CAD build for the part. Positions are in the model's coordinates, mm. A direction names the side the tool comes from. Coordinates: 2 decimals unless noted, no trailing zeros. Write each loop counter-clockwise with the first axis right and the second up, starting at its lowest first coordinate (ties: lowest second). Pieces come first, ordered by that corner, then holes. Notation, with made-up numbers: (14, 7) -> (24, 7) arc R5 ccw to (24, 13) -> close; hole circle Ø5 at (21.25, -37.5). An arc over 180 degrees is marked (long way). Answer as CSV lines item,"result". Start each with the question number.
```python
from build123d import *

# Parameters (mm, degrees)
BOSS_EXTRU_1_DEPTH      = 216
ENL_V_MAT_EXTRU_1_DEPTH = 49


with BuildPart() as part:
    # Esquisse1 → Boss.-Extru.1 (new body)
    with BuildSketch(Plane.XY):
        Polygon((105.75, 119), (105.75, 94), (80.75, 94), (80.75, 102), (57.75, 102), (57.75, 119), align=None)
    extrude(amount=BOSS_EXTRU_1_DEPTH)

    # Esquisse3 → Enlèv. mat.-Extru.1 (cut, through all)
    with BuildSketch(Plane(origin=(105.75, 0, 0), x_dir=(0, 0, -1), z_dir=(1, 0, 0))):
        Polygon((0, 119), (-25, 94), (0, 94), align=None)
        Polygon((-191, 94), (-216, 94), (-216, 119), align=None)
    extrude(amount=-ENL_V_MAT_EXTRU_1_DEPTH, mode=Mode.SUBTRACT)


solid = part.part
```
1. Cut at A-A (z = 83). Give the cut face in (x, y), then the cut area to 3 significant figures.
2. Tool access for faces 1 (the face through (80.75, 98, 107)), 2 (the face through (93, 94, 107)): list every direction of +Z, -Z, +X, -X, +Y, -Y with a clear straight run to the whole face (end or side of a thin tool).
3. Cut at B-B (y = 100). Give the cut face in (x, z), then the cut area to 3 significant figures.
4. Flat gauge pins, fed straight in: P1, Ø4, axis at x = 88.5, z = 193.5, coming from the -Y side; P2, Ø1, axis at x = 75, y = 107.5, coming from the +Z side; P3, Ø10, axis at x = 97, y = 100, coming from the -Z side. Where does each tip first touch, or does it go through?
5. Cut at C-C (x = 68.5). Give the cut face in (y, z).
6. Wall check: line 1 (Y direction, x = 77, z = 72); line 2 (X direction, y = 100.25, z = 31); line 3 (Z direction, x = 82, y = 96). Give the ranges that are in metal, low to high.
Geometry check:
1,outline,"(57.75, 102) -> (80.75, 102) -> (80.75, 94) -> (105.75, 94) -> (105.75, 119) -> (57.75, 119) -> close"
1,area,"1,020 mm²"
2,face 1,"+Z, -Z, -X, -Y"
2,face 2,"+Z, -Z, +X, -X, -Y"
3,outline,"(80.75, 19) -> (105.75, 19) -> (105.75, 197) -> (80.75, 197) -> close"
3,area,"4,450 mm²"
4,P1,"y = 94.5"
4,P2,"z = 205"
4,P3,"z = 14"
5,outline,"(102, 17) -> (119, 0) -> (119, 216) -> (102, 199) -> close"
6,line 1,"102 to 119"
6,line 2,"80.75 to 105.75"
6,line 3,"23 to 193"
